from build123d import *

# Parameters (mm, degrees)
F1_DEPTH = 10.922
F2_DEPTH = 22.352
F3_DEPTH = 38.354


with BuildPart() as f1:
    # F0 (on Top) → F1 (new body)
    with BuildSketch(Plane.XY):
        Polygon((-132.1051865816, 51.4431856573), (-132.1051865816, -10.2472146973), (-24.0534823388, 45.6737391651), align=None)
    extrude(amount=F1_DEPTH)

    # F2 (add): a face of the model
    f2_faces = [f1.faces().sort_by_distance(p)[0] for p in [
        (-78.0793344602, 17.7132622339, 5.461),
    ]]
    extrude(f2_faces, amount=F2_DEPTH)

    # F3 (add): a face of the model
    f3_faces = [f1.faces().sort_by_distance(p)[0] for p in [
        (-18.9166426466, 35.7482238648, 5.461),
    ]]
    extrude(f3_faces, amount=F3_DEPTH)


solid = f1.part
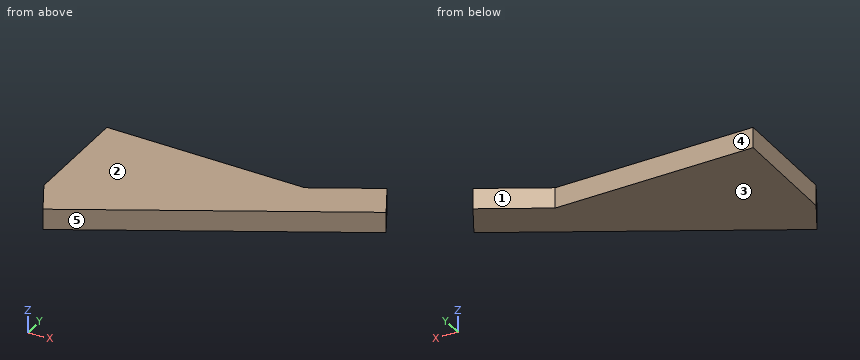
Model file for the job. Use its own axes, mm. Face numbers are marked on the shaded views. A direction names the side the tool comes from. Coordinates: 2 decimals unless noted, no trailing zeros. Loops run counter-clockwise (first coordinate to the right, second up) from the corner with the lowest first, then second, coordinate; pieces in that order, holes last. Notation, with made-up numbers: (-2, 31.5) -> (23, 31.5) arc R20 ccw to (23, 66.5) -> close; hole circle Ø3 at (8.25, -22). An arc over 180 degrees is marked (long way). Use one line per item in the form item = value. Start each with the question number.
(1) Cut at B-B on z = 7. Give the cut face in (x, y).
(2) Cut at D-D on y = 3.5. Give the cut face in (x, z), and give its area (3 significant figures).
(3) Pull direction X, two halves, no side cores. Call the marked faces 3, 4 and 5: pulls with the +X half, pulls with the -X half, needs draft (parallel to the pull), parting line crosses it, or undercut.
(4) Cut at A-A on y = 48. Give the cut face in (x, z).
(5) Cut at C-C on x = -86. Give the cut face in (y, z), and give its area (3 significant figures).
(6) Flat gauge pins, fed straight in: pin 1 (5 mm diameter, centred on x = -110, z = 4.5, fed in from -Y); pin 2 (6 mm diameter, centred on x = 1.5, z = 3.5, fed in from -Y); pin 3 (1.5 mm diameter, centred on y = 19, z = 5.5, fed in from +X). Where does each tip first touch, or does it go through?
(7) Probe probe 1 along X at (y, z) = (-9.5, 5.25); probe 2 along X at (y, z) = (38, 10.25); probe 3 along Y at (x, z) = (-28, 8.25). List the from-to ranges inside material, lowest first. Write a range as from..to.
(8) Tool access for the marked faces 1 and 2: list every direction of +Z, -Z, +X, -X, +Y, -Y with a clear straight run to the whole face (end or side of a thin tool).
Values:
q1.outline = (-132.11, -10.25) -> (-121.83, -30.1) -> (20.28, 43.45) -> (10.01, 63.3) -> (-24.05, 45.67) -> (-132.11, 51.44) -> close
q2.outline = (-132.11, 0) -> (-56.91, 0) -> (-56.91, 10.92) -> (-132.11, 10.92) -> close
q2.area = 821 mm2
q3.face_3 = needs draft
q3.face_4 = undercut
q3.face_5 = pulls with the +X half
q4.outline = (-132.11, 0) -> (-67.62, 0) -> (-67.62, 10.92) -> (-132.11, 10.92) -> close; (-19.56, 0) -> (17.93, 0) -> (17.93, 10.92) -> (-19.56, 10.92) -> close
q5.outline = (-11.55, 0) -> (48.98, 0) -> (48.98, 10.92) -> (-11.55, 10.92) -> close
q5.area = 661 mm2
q6.pin_1 = -25.27
q6.pin_2 = 32.18
q6.pin_3 = -25.51
q7.probe_1 = -132.11..-82.03
q7.probe_2 = -132.11..9.75
q7.probe_3 = 18.46..45.88
q8.face_1 = +Z, -Z, +Y
q8.face_2 = +Z, +X, -X, +Y, -Y
